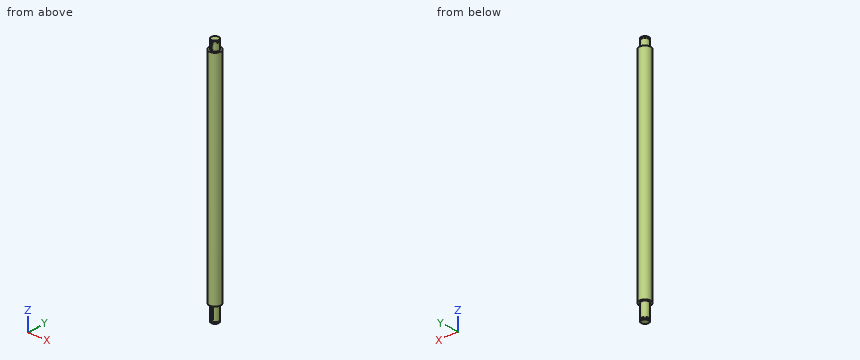
Autodesk Inventor part; units mm, degrees
ref_plane "工作平面1" through (0, -10, 280.932) normal (0, 1, 0) x (-1, 0, 0)
ref_plane "YZ Plane" through (0, 0, 0) normal (1, 0, 0) x (0, 1, 0)
ref_plane "XY Plane" through (0, 0, 0) normal (0, 0, 1) x (1, 0, 0)
sketch "草图1" plane through (0, 0, 0) normal (0, 0, 1) x (1, 0, 0)
  circle A0 centre (0, 0) radius 15
  dimension "d0" = 30
extrude "拉伸1" add sketch "草图1" along normal mid plane 561.864
sketch "草图2" plane through (0, 0, 280.932) normal (0, 0, 1) x (1, 0, 0)
  circle A0 centre (0, 0) radius 10
  dimension "d3" = 20
extrude "拉伸2" add sketch "草图2" along normal blind 23.97
ref_plane "工作平面1" through (0, -10, 280.932) normal (0, 1, 0) x (-1, 0, 0)
sketch "草图3" plane through (0, -10, 280.932) normal (0, 1, 0) x (-1, 0, 0)
  line L0 (-3, 13.385) -> (3, 13.385)
  line L1 (3, 13.385) -> (3, 5.385)
  line L2 (3, 5.385) -> (-3, 5.385)
  line L3 (-3, 5.385) -> (-3, 13.385)
  arc A0 (3, 13.385) -> (-3, 13.385) centre (0, 13.385) ccw
  arc A1 (-3, 5.385) -> (3, 5.385) centre (0, 5.385) ccw
  line L4 (15, 0) -> (-15, 0)
  line L5 (0, 0) -> (0, 30.5075)
  point P0 (0, -280.932)
  dimension "d6" = 30.5075
  dimension "d7" = 6
  dimension "d8" = 8
  dimension "d9" = 5.385
extrude "拉伸3" cut sketch "草图3" along normal blind 2.5
sketch "草图4" plane through (0, 0, 0) normal (0, 1, 0) x (-1, 0, 0)
  line L0 (-9.175, 299.702) -> (-11.2925, 299.702)
  line L1 (-11.2925, 299.702) -> (-11.2925, 300.902)
  line L2 (-11.2925, 300.902) -> (-9.175, 300.902)
  line L3 (-9.175, 300.902) -> (-9.175, 299.702)
  line L4 (0, 0) -> (0, 472.2352)
  line L5 (10, 304.902) -> (-10, 304.902)
  line L6 (0, -94.447) -> (0, 566.6823)
  dimension "d12" = 472.2352
  dimension "d13" = 9.175
  dimension "d14" = 1.2
  dimension "d15" = 4
  dimension "d16" = 2.1175
revolve "旋转1" cut sketch "草图4" angle 360 about axis through (0, 0, -10) along (0, 0, 1)
chamfer "倒角1" distance 0.5 angle 45 1 edges at (-10, 0, 304.902)
sketch "草图5" plane through (0, 0, -280.932) normal (0, 0, -1) x (-1, 0, 0)
  circle A0 centre (0, 0) radius 10
  dimension "d21" = 20
extrude "拉伸4" add sketch "草图5" along normal blind 41.61
sketch "草图6" plane through (0, -10, 280.932) normal (0, 1, 0) x (-1, 0, 0)
  line L0 (3, -593.069) -> (-3, -593.069)
  line L1 (-3, -593.069) -> (-3, -567.069)
  line L2 (-3, -567.069) -> (3, -567.069)
  line L3 (3, -567.069) -> (3, -593.069)
  arc A0 (-3, -593.069) -> (3, -593.069) centre (0, -593.069) ccw
  arc A1 (3, -567.069) -> (-3, -567.069) centre (0, -567.069) ccw
  line L4 (-10, -603.474) -> (10, -603.474)
  line L5 (0, -603.474) -> (0, -655.1956)
  line L6 (-15, -561.864) -> (15, -561.864)
  point P0 (0, -280.932)
  dimension "d24" = 6
  dimension "d25" = 26
  dimension "d26" = 5.205
extrude "拉伸5" cut sketch "草图6" along normal blind 2.5
sketch "草图7" plane through (0, 0, 0) normal (0, 1, 0) x (-1, 0, 0)
  line L0 (14.9872, -318.542) -> (9.175, -318.542)
  line L1 (9.175, -318.542) -> (9.175, -317.342)
  line L2 (9.175, -317.342) -> (14.9872, -317.342)
  line L3 (14.9872, -317.342) -> (14.9872, -318.542)
  line L4 (-10, -322.542) -> (10, -322.542)
  line L5 (0, -322.542) -> (0, -326.842)
  point P0 (0, 0)
  dimension "d29" = 4.3
  dimension "d30" = 1.2
  dimension "d31" = 5.8122
  dimension "d32" = 4
  dimension "d33" = 9.175
revolve "旋转2" cut sketch "草图7" angle 360 about axis through (0, 0, -322.542) along (0, 0, -1)
chamfer "倒角2" distance 1 angle 45 1 edges at (10, 0, -322.542)
properties part number "中间传动轴"
Geometry check sheet. Reference: the model listing, model coordinates, mm. Coordinates: 2 decimals unless noted, no trailing zeros. Order: outer loops, then holes, each group sorted by start corner. A loop starts at its lowest first (then second) coordinate and runs counter-clockwise, first axis right, second up. Notation, with made-up numbers: M 17.5,79.25 L 46.5,79.25 A16 cw 46.5,95.25 Z; hole C 56,41 d9. An arc over 180 degrees is marked long. Use CSV: the item, a comma, the result in double quotes.
Item 1: Thickness scan on line 1 along Y through (x, z) = (1.5, -21.5); line 2 along X through (y, z) = (1, 12.5); line 3 along Y through (x, z) = (0.25, 113.5). Record the ranges inside material, lowest first.
Returned:
line 1,"y = -14.92 to 14.92"
line 2,"x = -14.97 to 14.97"
line 3,"y = -15 to 15"
Item 2: Cross-section at B-B on z = -119. Record the cut outline in (x, y).
Returned:
outline,"C 0,0 d30"
Item 3: Gauge pin test, flat ends, axial feed: pin 1 Ø1 at (y, z) = (-8.5, 289.5) entering from -X; pin 2 Ø3 at (x, z) = (0.5, 288) entering from -Y; pin 3 Ø2 at (y, z) = (-8, 76.5) entering from +X. Record the tip position at first contact, or that the pin passes through.
Returned:
pin 1,"stops at x = -6"
pin 2,"stops at y = -7.5"
pin 3,"stops at x = 13.27"
